from build123d import *

# Parameters (mm, degrees)
BOSS_EXTRUDE3_DEPTH  = 12
BOSS_EXTRUDE5_DEPTH  = 12
BOSS_EXTRUDE6_DEPTH  = 12
BOSS_EXTRUDE7_DEPTH  = 12
SKETCH13_W           = 102
SKETCH13_H           = 12
BOSS_EXTRUDE11_DEPTH = 1
SKETCH14_W           = 103
SKETCH14_H           = 12
BOSS_EXTRUDE12_DEPTH = 1
SKETCH15_W           = 103
SKETCH15_H           = 12
BOSS_EXTRUDE13_DEPTH = 1
SKETCH16_W           = 104
SKETCH16_H           = 12
BOSS_EXTRUDE14_DEPTH = 1
SKETCH17_W           = 104
SKETCH17_H           = 104
BOSS_EXTRUDE16_DEPTH = 12
SKETCH20_W           = 104
SKETCH20_H           = 24
BOSS_EXTRUDE20_DEPTH = 10
CUT_EXTRUDE2_DEPTH   = 104
SKETCH23_W           = 104
SKETCH23_H           = 24
BOSS_EXTRUDE21_DEPTH = 10
CUT_EXTRUDE3_DEPTH   = 104
SKETCH26_W           = 10.4
SKETCH26_H           = 41.4
SKETCH26_W_2         = 10
SKETCH26_H_2         = 41
CUT_EXTRUDE5_DEPTH   = 7.5
SKETCH29_W           = 5
SKETCH29_H           = 104
CUT_EXTRUDE6_DEPTH   = 8
SKETCH30_W           = 5
SKETCH30_H           = 104
CUT_EXTRUDE7_DEPTH   = 8
BOSS_EXTRUDE22_DEPTH = 5
SKETCH33_W           = 41.4
SKETCH33_H           = 7.5
BOSS_EXTRUDE23_DEPTH = 5
BOSS_EXTRUDE24_DEPTH = 5
SKETCH35_W           = 41
SKETCH35_H           = 7.5
BOSS_EXTRUDE25_DEPTH = 5
SKETCH36_R           = 1.5
CUT_EXTRUDE8_DEPTH   = 2.5
SKETCH37_R           = 1.5
CUT_EXTRUDE9_DEPTH   = 2.5
SKETCH38_R           = 2.5
SKETCH38_R_2         = 1.5
BOSS_EXTRUDE26_DEPTH = 10


with BuildPart() as part:
    # Sketch1 → Boss-Extrude3 (new body)
    with BuildSketch(Plane(origin=(0, 0, 0), x_dir=(1, 0, 0), z_dir=(0, 1, 0))):
        with BuildLine():
            Line((-46, 51), (46, 51))
            ThreePointArc((46, 51), (49.535533906, 49.535533906), (51, 46))
            Line((51, 46), (51, -46))
            ThreePointArc((51, -46), (49.535533906, -49.535533906), (46, -51))
            Line((46, -51), (-46, -51))
            ThreePointArc((-46, -51), (-49.535533906, -49.535533906), (-51, -46))
            Line((-51, -46), (-51, 46))
            ThreePointArc((-51, 46), (-49.535533906, 49.535533906), (-46, 51))
        make_face()
    extrude(amount=BOSS_EXTRUDE3_DEPTH)

    # Sketch4 → Boss-Extrude5 (add)
    with BuildSketch(Plane(origin=(0, 0, 0), x_dir=(-1, 0, 0), z_dir=(0, -1, 0))):
        with BuildLine():
            Line((-46, -51), (-51, -51))
            Line((-51, -51), (-51, -46))
            ThreePointArc((-51, -46), (-49.535533906, -49.535533906), (-46, -51))
        make_face()
    extrude(amount=-BOSS_EXTRUDE5_DEPTH)

    # Sketch6 → Boss-Extrude6 (add)
    with BuildSketch(Plane.XZ):
        with BuildLine():
            Line((-51, -46), (-51, -51))
            Line((-51, -51), (-46, -51))
            ThreePointArc((-46, -51), (-49.535533906, -49.535533906), (-51, -46))
        make_face()
    extrude(amount=-BOSS_EXTRUDE6_DEPTH)

    # Sketch7 → Boss-Extrude7 (add)
    with BuildSketch(Plane.XZ):
        with BuildLine():
            Line((-46, 51), (-51, 51))
            Line((-51, 51), (-51, 46))
            ThreePointArc((-51, 46), (-49.535533906, 49.535533906), (-46, 51))
        make_face()
        with BuildLine():
            Line((46, -51), (51, -51))
            Line((51, -51), (51, -46))
            ThreePointArc((51, -46), (49.535533906, -49.535533906), (46, -51))
        make_face()
    extrude(amount=-BOSS_EXTRUDE7_DEPTH)

    # Sketch13 → Boss-Extrude11 (add)
    with BuildSketch(Plane.XY.offset(51)):
        with Locations((0, 6)):
            Rectangle(SKETCH13_W, SKETCH13_H)
    extrude(amount=BOSS_EXTRUDE11_DEPTH)

    # Sketch14 → Boss-Extrude12 (add)
    with BuildSketch(Plane(origin=(51, 0, 0), x_dir=(0, 0, -1), z_dir=(1, 0, 0))):
        with Locations((-0.5, 6)):
            Rectangle(SKETCH14_W, SKETCH14_H)
    extrude(amount=BOSS_EXTRUDE12_DEPTH)

    # Sketch15 → Boss-Extrude13 (add)
    with BuildSketch(Plane(origin=(0, 0, -51), x_dir=(-1, 0, 0), z_dir=(0, 0, -1))):
        with Locations((-0.5, 6)):
            Rectangle(SKETCH15_W, SKETCH15_H)
    extrude(amount=BOSS_EXTRUDE13_DEPTH)

    # Sketch16 → Boss-Extrude14 (add)
    with BuildSketch(Plane.ZY.offset(51)):
        with Locations((0, 6)):
            Rectangle(SKETCH16_W, SKETCH16_H)
    extrude(amount=BOSS_EXTRUDE14_DEPTH)

    # Sketch17 → Boss-Extrude16 (add)
    with BuildSketch(Plane(origin=(0, 12, 0), x_dir=(1, 0, 0), z_dir=(0, 1, 0))):
        Rectangle(SKETCH17_W, SKETCH17_H)
        with BuildLine():
            Line((-45, 50), (45, 50))
            ThreePointArc((45, 50), (48.535533906, 48.535533906), (50, 45))
            Line((50, 45), (50, -45))
            ThreePointArc((50, -45), (48.535533906, -48.535533906), (45, -50))
            Line((45, -50), (-45, -50))
            ThreePointArc((-45, -50), (-48.535533906, -48.535533906), (-50, -45))
            Line((-50, -45), (-50, 45))
            ThreePointArc((-50, 45), (-48.535533906, 48.535533906), (-45, 50))
        make_face(mode=Mode.SUBTRACT)
    extrude(amount=BOSS_EXTRUDE16_DEPTH)

    # Sketch20 → Boss-Extrude20 (add)
    with BuildSketch(Plane(origin=(52, 0, 0), x_dir=(0, 0, -1), z_dir=(1, 0, 0))):
        with Locations((0, 12)):
            Rectangle(SKETCH20_W, SKETCH20_H)
    extrude(amount=BOSS_EXTRUDE20_DEPTH)

    # Sketch21 → Cut-Extrude2 (cut)
    with BuildSketch(Plane.XY.offset(52)):
        Polygon((62, 24), (52, 24), (57, 18), (62, 18), align=None)
    extrude(amount=-CUT_EXTRUDE2_DEPTH, mode=Mode.SUBTRACT)

    # Sketch23 → Boss-Extrude21 (add)
    with BuildSketch(Plane.ZY.offset(52)):
        with Locations((0, 12)):
            Rectangle(SKETCH23_W, SKETCH23_H)
    extrude(amount=BOSS_EXTRUDE21_DEPTH)

    # Sketch24 → Cut-Extrude3 (cut)
    with BuildSketch(Plane.XY.offset(52)):
        Polygon((-62, 24), (-52, 24), (-57, 18), (-62, 18), align=None)
    extrude(amount=-CUT_EXTRUDE3_DEPTH, mode=Mode.SUBTRACT)

    # Sketch26 → Cut-Extrude5 (cut)
    with BuildSketch(Plane.XZ):
        with Locations((-56.8, 0)):
            Rectangle(SKETCH26_W, SKETCH26_H)
        with Locations((57, 0)):
            Rectangle(SKETCH26_W_2, SKETCH26_H_2)
    extrude(amount=-CUT_EXTRUDE5_DEPTH, mode=Mode.SUBTRACT)

    # Sketch29 → Cut-Extrude6 (cut)
    with BuildSketch(Plane(origin=(0, 18, 0), x_dir=(1, 0, 0), z_dir=(0, 1, 0))):
        with Locations((59.5, 0)):
            Rectangle(SKETCH29_W, SKETCH29_H)
    extrude(amount=-CUT_EXTRUDE6_DEPTH, mode=Mode.SUBTRACT)

    # Sketch30 → Cut-Extrude7 (cut)
    with BuildSketch(Plane(origin=(0, 18, 0), x_dir=(1, 0, 0), z_dir=(0, 1, 0))):
        with Locations((-59.5, 0)):
            Rectangle(SKETCH30_W, SKETCH30_H)
    extrude(amount=-CUT_EXTRUDE7_DEPTH, mode=Mode.SUBTRACT)

    # Sketch32 → Boss-Extrude22 (add)
    with BuildSketch(Plane.ZY.offset(62)):
        Polygon((-52, 10), (-52, 0), (-20.7, 0), (-20.7, 7.5), (20.7, 7.5), (20.7, 0), (52, 0), (52, 10), align=None)
    extrude(amount=BOSS_EXTRUDE22_DEPTH)

    # Sketch33 → Boss-Extrude23 (add)
    with BuildSketch(Plane.ZY.offset(51.6)):
        with Locations((0, 3.75)):
            Rectangle(SKETCH33_W, SKETCH33_H)
    extrude(amount=BOSS_EXTRUDE23_DEPTH)

    # Sketch34 → Boss-Extrude24 (add)
    with BuildSketch(Plane(origin=(62, 0, 0), x_dir=(0, 0, -1), z_dir=(1, 0, 0))):
        Polygon((-52, 10), (-52, 0), (-20.5, 0), (-20.5, 7.5), (20.5, 7.5), (20.5, 0), (52, 0), (52, 10), align=None)
    extrude(amount=BOSS_EXTRUDE24_DEPTH)

    # Sketch35 → Boss-Extrude25 (add)
    with BuildSketch(Plane(origin=(52, 0, 0), x_dir=(0, 0, -1), z_dir=(1, 0, 0))):
        with Locations((0, 3.75)):
            Rectangle(SKETCH35_W, SKETCH35_H)
    extrude(amount=BOSS_EXTRUDE25_DEPTH)

    # Sketch36 → Cut-Extrude8 (cut)
    with BuildSketch(Plane.XZ.offset(-7.5)):
        with Locations((62, 12)):
            Circle(SKETCH36_R)
        with Locations((62, -12)):
            Circle(SKETCH36_R)
    extrude(amount=-CUT_EXTRUDE8_DEPTH, mode=Mode.SUBTRACT)

    # Sketch37 → Cut-Extrude9 (cut)
    with BuildSketch(Plane.XZ.offset(-7.5)):
        with Locations((-62, 12)):
            Circle(SKETCH37_R)
        with Locations((-62, -12)):
            Circle(SKETCH37_R)
    extrude(amount=-CUT_EXTRUDE9_DEPTH, mode=Mode.SUBTRACT)

    # Sketch38 → Boss-Extrude26 (add)
    with BuildSketch(Plane(origin=(0, 12, 0), x_dir=(1, 0, 0), z_dir=(0, 1, 0))):
        with BuildLine():
            Line((-42.5, 50), (-45, 50))
            ThreePointArc((-45, 50), (-48.535533906, 48.535533906), (-50, 45))
            Line((-50, 45), (-50, 42.5))
            Line((-50, 42.5), (-45, 42.5))
            ThreePointArc((-45, 42.5), (-46.767766953, 46.767766953), (-42.5, 45))
            Line((-42.5, 45), (-42.5, 50))
        make_face()
        with Locations((-45, 45)):
            Circle(SKETCH38_R)
        with Locations((-45, 45)):
            Circle(SKETCH38_R_2, mode=Mode.SUBTRACT)
        with BuildLine():
            Line((45, 50), (42.5, 50))
            Line((42.5, 50), (42.5, 45))
            ThreePointArc((42.5, 45), (45, 47.5), (47.5, 45))
            ThreePointArc((47.5, 45), (46.767766953, 43.232233047), (45, 42.5))
            Line((45, 42.5), (50, 42.5))
            Line((50, 42.5), (50, 45))
            ThreePointArc((50, 45), (48.535533906, 48.535533906), (45, 50))
        make_face()
        with Locations((45, 45)):
            Circle(SKETCH38_R)
        with Locations((45, 45)):
            Circle(SKETCH38_R_2, mode=Mode.SUBTRACT)
        with BuildLine():
            Line((-45, -42.5), (-50, -42.5))
            Line((-50, -42.5), (-50, -45))
            ThreePointArc((-50, -45), (-48.535533906, -48.535533906), (-45, -50))
            Line((-45, -50), (-42.5, -50))
            Line((-42.5, -50), (-42.5, -45))
            ThreePointArc((-42.5, -45), (-46.767766953, -46.767766953), (-45, -42.5))
        make_face()
        with Locations((-45, -45)):
            Circle(SKETCH38_R)
        with Locations((-45, -45)):
            Circle(SKETCH38_R_2, mode=Mode.SUBTRACT)
        with BuildLine():
            Line((50, -45), (50, -42.5))
            Line((50, -42.5), (45, -42.5))
            ThreePointArc((45, -42.5), (46.767766953, -43.232233047), (47.5, -45))
            ThreePointArc((47.5, -45), (45, -47.5), (42.5, -45))
            Line((42.5, -45), (42.5, -50))
            Line((42.5, -50), (45, -50))
            ThreePointArc((45, -50), (48.535533906, -48.535533906), (50, -45))
        make_face()
        with Locations((45, -45)):
            Circle(SKETCH38_R)
        with Locations((45, -45)):
            Circle(SKETCH38_R_2, mode=Mode.SUBTRACT)
    extrude(amount=BOSS_EXTRUDE26_DEPTH)


solid = part.part
The model under review builds one solid part; all positions refer to its coordinate system, in mm. A direction names the side the tool comes from. Coordinates: 2 decimals unless noted, no trailing zeros. Loops run counter-clockwise (first coordinate to the right, second up) from the corner with the lowest first, then second, coordinate; pieces in that order, holes last. Notation, with made-up numbers: M -4.75,83 L 4.25,83 A13 cw 4.25,93 Z; hole C -28,33.25 d9. An arc over 180 degrees is marked long. Put each result on its own line as item: value. Start each with the question number.
Q1. The part is to be moulded in two halves that separate along X. For faces 4 (the flat face through (45, 12, -45)), 5 (the flat face through (-1, 12, 52)), 6 (the flat face through (57, 14, 1)), 7 (the cylindrical face through (63.43, 8.73, -11.55)), say which applies: +X half, -X half, draft (parallel to the pull), parting line (faces both ways), or undercut.
Q2. Add section D-D (x = 34). Write out the cut boundary in (y, z).
Q3. Add section B-B (x = 62). Write out the cut boundary in (y, z), and give its area (4 significant figures).
Q4. Wall thickness on line 1 (Z direction, x = -45, y = 14.75); line 2 (Z direction, x = -62, y = 9.5); line 3 (X direction, y = 17, z = 45): over which ranges is each line inside the solid? List them lowest first.
Q5. Clearance check with flat-ended pins moving along their axes: pin 1 (1.5 mm diameter, centred on x = 45.5, z = -44.5, fed in from +Y); pin 2 (13 mm diameter, centred on y = 20.5, z = -11.5, fed in from -X); pin 3 (11.5 mm diameter, centred on x = -63, z = -3.5, fed in from -Y). State where each tip first meets the part, or that it passes through.
Q6. Add section C-C (y = 15). Write out the cut boundary in (x, z).
Q7. For faces 1 (the flat face through (-62, 10, 1)), 2 (the flat face through (57, 4, 0)), 3 (the flat face through (-50, 18, 1)), list the 3-axis set-ups (+Z, -Z, +X, -X, +Y, -Y) from which the entire face can be reached by the end or side of a thin tool; tool diameter is ignored.
Q8. Add section A-A (z = -12). Write out the cut boundary in (x, y).
Answers:
1. face 4: undercut
1. face 5: draft
1. face 6: +X half
1. face 7: undercut
2. outline: M 0,-52 L 24,-52 L 24,-50 L 12,-50 L 12,50 L 24,50 L 24,52 L 0,52 Z
3. outline: M 0,-52 L 10,-52 L 10,-13.5 L 7.5,-13.5 L 7.5,-20.5 L 0,-20.5 Z; M 0,20.5 L 7.5,20.5 L 7.5,13.5 L 10,13.5 L 10,52 L 0,52 Z; M 7.5,-10.5 L 10,-10.5 L 10,10.5 L 7.5,10.5 Z
3. area: 717.5 mm^2
4. line 1: z = -52 to -46.5, -43.5 to -42.5, 42.5 to 43.5, 46.5 to 52
4. line 2: z = -52 to -13.5, -10.5 to 10.5, 13.5 to 52
4. line 3: x = -57 to -46.5, -43.5 to -42.5, 42.5 to 43.5, 46.5 to 57
5. pin 1: stops at y = 12
5. pin 2: stops at x = -57
5. pin 3: stops at y = 7.5
6. outline: M -57,-52 L 57,-52 L 57,52 L -57,52 Z; hole M -50,-42.5 L -45,-42.5 A2.5 cw -42.5,-45 L -42.5,-50 L 42.5,-50 L 42.5,-45 A2.5 cw 45,-42.5 L 50,-42.5 L 50,42.5 L 45,42.5 A2.5 cw 42.5,45 L 42.5,50 L -42.5,50 L -42.5,45 A2.5 cw -45,42.5 L -50,42.5 Z; hole C -45,-45 d3; hole C -45,45 d3; hole C 45,-45 d3; hole C 45,45 d3
7. face 1: +Z, -Z, -X, +Y
7. face 2: +X, -Y
7. face 3: +Y
8. outline: M -67,7.5 L -63.5,7.5 L -63.5,10 L -67,10 Z; M -60.5,7.5 L -56.6,7.5 L -56.6,0 L 57,0 L 57,7.5 L 60.5,7.5 L 60.5,10 L 57,10 L 57,18 L 52,24 L 50,24 L 50,12 L -50,12 L -50,24 L -52,24 L -57,18 L -57,10 L -60.5,10 Z; M 63.5,7.5 L 67,7.5 L 67,10 L 63.5,10 Z
